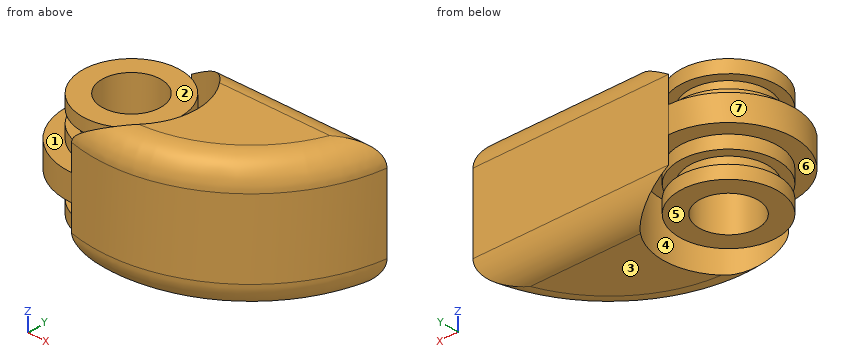
Autodesk Inventor part; units mm, degrees
ref_plane "YZ Plane" through (0, 0, 0) normal (1, 0, 0) x (0, 1, 0)
ref_plane "XZ Plane" through (0, 0, 0) normal (0, 1, 0) x (-1, 0, 0)
ref_plane "XY Plane" through (0, 0, 0) normal (0, 0, 1) x (1, 0, 0)
sketch "Sketch1" plane through (0, 0, 0) normal (0, 0, 1) x (1, 0, 0)
  circle A0 centre (0, 0) radius 10
  line L0 (0, 10) -> (30, 10)
  arc A1 (0, -10) -> (30, 10) centre (6.2119, 13.1822) ccw
  circle A2 centre (0, 0) radius 4.5
  circle A3 centre (0, 0) radius 7.5
  circle A4 centre (0, 0) radius 6
  dimension "d0" = 20
  dimension "d1" = 30
  dimension "d2" = 24
  dimension "d3" = 10
  dimension "d4" = 13.1822
  dimension "d5" = 9
  dimension "d6" = 15
  dimension "d7" = 12
extrude "Extrusion1" add sketch "Sketch1" along normal mid plane 20 contours A0 L0 A1
extrude "Extrusion2" add sketch "Sketch1" along normal mid plane 4 contours A0 | A3 | A4
extrude "Extrusion3" add sketch "Sketch1" along normal mid plane 8 contours A3 | A4
extrude "Extrusion4" add sketch "Sketch1" along normal mid plane 12 contours A4
sketch "Sketch2" plane through (0, 0, 6) normal (0, 0, 1) x (1, 0, 0)
  circle A0 centre (0, 0) radius 7.5
  circle A1 centre (0, 0) radius 4.5
  dimension "d16" = 15
  dimension "d18" = 9
sketch "Sketch3" plane through (0, 0, -6) normal (0, 0, -1) x (-1, 0, 0)
  circle A0 centre (0, 0) radius 7.5
  circle A1 centre (0, 0) radius 4.5
  dimension "d17" = 15
  dimension "d19" = 9
extrude "Extrusion5" add sketch "Sketch3" along normal blind 2
extrude "Extrusion6" add sketch "Sketch2" along normal blind 2
fillet "Fillet1" radius 4 4 edges at (15, 10, -10) (19.5247, -6.7871, -10) (19.5247, -6.7871, 10) (15, 10, 10)
properties part number "TapPart"
Work out the finished part from the listing and answer in its coordinate system (mm). Face numbers are marked on the shaded views. A direction names the side the tool comes from. Coordinates: 2 decimals unless noted, no trailing zeros. Write each loop counter-clockwise with the first axis right and the second up, starting at its lowest first coordinate (ties: lowest second). Pieces come first, ordered by that corner, then holes. Notation, with made-up numbers: M 51.5,7.5 L 72.5,7.5 A19 cw 72.5,16.5 Z; hole C 52.5,-7.75 d11. An arc over 180 degrees is marked long. Answer as CSV lines item,"result". Start each with the question number.
Item 1: Determine the mould class of the marked faces 4, 5, 6 and 7 for opening direction X: released by +X, released by -X, zero draft, split by the parting line, or undercut.
Item 2: Flat-ended cylindrical pins translate along their axes: P1, Ø10, axis at x = 2, y = 1, coming from the -Z side; P2, Ø4, axis at y = -8.5, z = 1.5, coming from the +X side; P3, Ø10, axis at x = 3.5, y = 3, coming from the +Z side. Find the tip coordinate at first contact, or state that the pin passes through.
Item 3: Consider L1, parallel to Z at x = 7, y = -0.75; L2, parallel to Y at x = 0, z = -0.25; L3, parallel to X at y = 0.25, z = -7.25. Determine where each line is inside the solid, lowest interval first.
Item 4: A tool of negligible diameter and unlimited length cuts with its end or side. For the marked faces 1, 2 and 3, from which of +Z, -Z, +X, -X, +Y, -Y can it reach the whole face along a straight path? Write none if from no direction.
Item 5: Section A-A on z = -5.25 is taken. Write down the section's boundary in (x, y), and give its area (3 significant figures).
Item 6: Section C-C on z = -1 is taken. Write down the section's boundary in (x, y), and give its area (3 significant figures).
Item 7: Section B-B on z = 3.25 is taken. Write down the section's boundary in (x, y).
Checks:
1,face 4,"undercut"
1,face 5,"zero draft"
1,face 6,"undercut"
1,face 7,"released by -X"
2,P1,"stops at z = -8"
2,P2,"stops at x = 19.95"
2,P3,"stops at z = 8"
3,L1,"z = -8 to -6, -4 to 4, 6 to 8"
3,L2,"y = -10 to -4.5, 4.5 to 10"
3,L3,"x = -7.5 to -4.49, 4.49 to 7.5, 10 to 26.19"
4,face 1,"+Z"
4,face 2,"+Z, -X"
4,face 3,"-Z, +X, -X, +Y, -Y"
5,outline,"C 0,0 d12; M 0,-10 A24 ccw 30,10 L 0,10 A10 cw Z; hole C 0,0 d9"
5,area,"396 mm²"
6,outline,"M 0,-10 A24 ccw 30,10 L 0,10 A10 ccw Z; hole C 0,0 d9"
6,area,"597 mm²"
7,outline,"C 0,0 d15; M 0,-10 A24 ccw 30,10 L 0,10 A10 cw Z; hole C 0,0 d9"
